```python
from build123d import *

# Parameters (mm, degrees)
SZKIC1_W                    = 200
SZKIC1_H                    = 20
SZKIC1_R                    = 3
SZKIC1_R_2                  = 3.25
DODANIE_WYCI_GNI_CIE1_DEPTH = 7


with BuildPart() as part:
    # Szkic1 → Dodanie-wyciągnięcie1 (new body)
    with BuildSketch(Plane(origin=(0, 0, 0), x_dir=(1, 0, 0), z_dir=(0, 1, 0))):
        with Locations((100, 10)):
            Rectangle(SZKIC1_W, SZKIC1_H)
        with Locations(Location((100, 10, 0), (0, 0, 270))):
            Circle(SZKIC1_R, mode=Mode.SUBTRACT)
        with Locations(Location((10, 10, 0), (0, 0, 270))):
            Circle(SZKIC1_R_2, mode=Mode.SUBTRACT)
        with Locations(Location((190, 10, 0), (0, 0, 270))):
            Circle(SZKIC1_R_2, mode=Mode.SUBTRACT)
        with BuildLine():
            Line((22.984822323, 15.57457628), (86.25939238, 15.57457628))
            ThreePointArc((86.25939238, 15.57457628), (89.794926286, 14.110110186), (91.25939238, 10.57457628))
            Line((91.25939238, 10.57457628), (91.25939238, 9.696719379))
            ThreePointArc((91.25939238, 9.696719379), (89.794926286, 6.161185473), (86.25939238, 4.696719379))
            Line((86.25939238, 4.696719379), (22.984822323, 4.696719379))
            ThreePointArc((22.984822323, 4.696719379), (19.449288417, 6.161185473), (17.984822323, 9.696719379))
            Line((17.984822323, 9.696719379), (17.984822323, 10.57457628))
            ThreePointArc((17.984822323, 10.57457628), (19.449288417, 14.110110186), (22.984822323, 15.57457628))
        make_face(mode=Mode.SUBTRACT)
        with BuildLine():
            Line((113.225148066, 15.57457628), (176.286209663, 15.57457628))
            ThreePointArc((176.286209663, 15.57457628), (179.821743569, 14.110110186), (181.286209663, 10.57457628))
            Line((181.286209663, 10.57457628), (181.286209663, 9.752776346))
            ThreePointArc((181.286209663, 9.752776346), (179.821743569, 6.21724244), (176.286209663, 4.752776346))
            Line((176.286209663, 4.752776346), (113.225148066, 4.752776346))
            ThreePointArc((113.225148066, 4.752776346), (109.68961416, 6.21724244), (108.225148066, 9.752776346))
            Line((108.225148066, 9.752776346), (108.225148066, 10.57457628))
            ThreePointArc((108.225148066, 10.57457628), (109.68961416, 14.110110186), (113.225148066, 15.57457628))
        make_face(mode=Mode.SUBTRACT)
    extrude(amount=DODANIE_WYCI_GNI_CIE1_DEPTH)


solid = part.part
```
Work out the finished part from the listing and answer in its coordinate system (mm). A direction names the side the tool comes from. Give positions to 0.01 mm unless a question says otherwise; leave off trailing zeros. Loops run counter-clockwise (first coordinate to the right, second up) from the corner with the lowest first, then second, coordinate; pieces in that order, holes last. Notation, with made-up numbers: (-5, -18) -> (20, -18) arc R18 ccw to (20, -13) -> close; hole circle Ø5 at (-39.5, 10.5). An arc over 180 degrees is marked (long way). One line per question, with ' | ' between items. Start each with the question number.
1) Section A-A, the plane x = 100 is taken. Determine the outline of the cut face in (y, z), then the cut area to 3 significant figures.
2) Section B-B, the plane y = 2 is taken. Determine the outline of the cut face in (x, z), then the cut area to 3 significant figures.
3) Section C-C, the plane x = 123 is taken. Determine the outline of the cut face in (y, z), then the cut area to 3 significant figures.
4) This flat-tipped pin is pushed along its axis until it touches: pin 1 (4 mm diameter, centred on x = 190, z = -10, fed in from +Y). Where does it stop, or does it pass through?
5) For faces 1 (the face through (99, 3, 0)), 2 (the face through (145, 3, -4.753)), determine the directions among +Z, -Z, +X, -X, +Y, -Y from which every point of the face is accessible in a straight line to the end or side of a thin tool.
6) Determine the mould class of faces 3 (the face through (99, 3, -20)), 4 (the face through (55, 3, -4.697)), 5 (the face through (89.834, 3.451, -6.2)), 6 (the face through (200, 3, -10)) for opening direction X: +X half, -X half, draft (parallel to the pull), parting line (faces both ways), or undercut.
7) Straight lines are drawn through the part: L1, parallel to X at y = 4, z = -10; L2, parallel to Z at x = 66, y = 5; L3, parallel to X at y = 4, z = -10.75. For each, find the intervals that lie inside material, in ascending order.
Resolved:
1) outline: (0, -20) -> (7, -20) -> (7, -13) -> (0, -13) -> close; (0, -7) -> (7, -7) -> (7, 0) -> (0, 0) -> close | area: 98.0 mm2
2) outline: (0, -20) -> (200, -20) -> (200, 0) -> (0, 0) -> close; hole circle Ø6.5 at (10, -10); hole (17.98, -10.57) arc R5 ccw to (22.98, -15.57) -> (86.26, -15.57) arc R5 ccw to (91.26, -10.57) -> (91.26, -9.7) arc R5 ccw to (86.26, -4.7) -> (22.98, -4.7) arc R5 ccw to (17.98, -9.7) -> close; hole circle Ø6 at (100, -10); hole (108.23, -10.57) arc R5 ccw to (113.23, -15.57) -> (176.29, -15.57) arc R5 ccw to (181.29, -10.57) -> (181.29, -9.75) arc R5 ccw to (176.29, -4.75) -> (113.23, -4.75) arc R5 ccw to (108.23, -9.75) -> close; hole circle Ø6.5 at (190, -10) | area: 2,360 mm2
3) outline: (0, -20) -> (7, -20) -> (7, -15.57) -> (0, -15.57) -> close; (0, -4.75) -> (7, -4.75) -> (7, 0) -> (0, 0) -> close | area: 64.2 mm2
4) pin 1: through
5) face 1: +Z, +X, -X, +Y, -Y | face 2: +Y, -Y
6) face 3: draft | face 4: undercut | face 5: undercut | face 6: +X half
7) L1: 0 to 6.75, 13.25 to 17.98, 91.26 to 97, 103 to 108.23, 181.29 to 186.75, 193.25 to 200 | L2: -20 to -15.57, -4.7 to 0 | L3: 0 to 6.84, 13.16 to 17.99, 91.26 to 97.1, 102.9 to 108.23, 181.28 to 186.84, 193.16 to 200
